```python
from build123d import *

# Parameters (mm, degrees)
ESQUISSE1_W        = 100
ESQUISSE1_H        = 100
ESQUISSE1_R        = 1.6
BOSS_EXTRU_1_DEPTH = 1.6
ESQUISSE2_R        = 5
BOSS_EXTRU_2_DEPTH = 20
ESQUISSE3_W        = 27.619166331
ESQUISSE3_H        = 14.436937143
BOSS_EXTRU_3_DEPTH = 15


with BuildPart() as part:
    # Esquisse1 → Boss.-Extru.1 (new body)
    with BuildSketch(Plane.XY):
        Rectangle(ESQUISSE1_W, ESQUISSE1_H)
        with Locations((-46, 46)):
            Circle(ESQUISSE1_R, mode=Mode.SUBTRACT)
        with Locations((46, 46)):
            Circle(ESQUISSE1_R, mode=Mode.SUBTRACT)
        with Locations((46, 4)):
            Circle(ESQUISSE1_R, mode=Mode.SUBTRACT)
        with Locations((-46, 4)):
            Circle(ESQUISSE1_R, mode=Mode.SUBTRACT)
        with Locations((-46, -46)):
            Circle(ESQUISSE1_R, mode=Mode.SUBTRACT)
        with Locations((46, -46)):
            Circle(ESQUISSE1_R, mode=Mode.SUBTRACT)
    extrude(amount=BOSS_EXTRU_1_DEPTH)

    # Esquisse2 → Boss.-Extru.2 (add)
    with BuildSketch(Plane.XY.offset(1.6)):
        with Locations((-26.099103373, -42.842866213)):
            Circle(ESQUISSE2_R)
        with Locations((-10.063114572, -42.842866213)):
            Circle(ESQUISSE2_R)
        with Locations((41.376738419, -34.563702957)):
            Circle(ESQUISSE2_R)
    extrude(amount=BOSS_EXTRU_2_DEPTH)

    # Esquisse3 → Boss.-Extru.3 (add)
    with BuildSketch(Plane.XY.offset(1.6)):
        with Locations((-34.191305716, 27.512141018)):
            Rectangle(ESQUISSE3_W, ESQUISSE3_H)
    extrude(amount=BOSS_EXTRU_3_DEPTH)


solid = part.part
```
Input: part model. Units: mm. Frame: model coordinates. A direction names the side the tool comes from. Give positions to 0.01 mm unless a question says otherwise; leave off trailing zeros. Order: outer loops, then holes, each group sorted by start corner. A loop starts at its lowest first (then second) coordinate and runs counter-clockwise, first axis right, second up.
1. Reachability of faces 5 (the cylindrical face through (36.38, -34.34, 11.46)), 6 (the flat face through (-34, 28, 16.6)), 7 (the flat face through (-20.382, 27, 9)), 8 (the flat face through (-34, 20.294, 9)) from +Z, -Z, +X, -X, +Y, -Y: full face, straight path, thin tool, end or side. Return the list, or none.
Derived:
face 5: +Z
face 6: +Z, +X, -X, +Y
face 7: +Z, +X, +Y, -Y
face 8: +Z, +X, -X
2. Mould query, pull axis Y, two halves, no side actions, for faces 1 (the flat face through (-34, 34.731, 9)), 2 (the flat face through (-48.001, 27, 9)), 3 (the cylindrical face through (-7.8, -47.3, 11.5)), 4 (the cylindrical face through (-27.183, -47.724, 11.46)). Classes: released by +Y, released by -Y, zero draft, split by the parting line, or undercut.
Derived:
face 1: released by +Y
face 2: zero draft
face 3: split by the parting line
face 4: undercut
3. Section A-A on y = 46. Return the cut outline in (x, z), and give its area (3 significant figures).
Derived:
outline: (-50, 0) - (-47.6, 0) - (-47.6, 1.6) - (-50, 1.6) - close; (-44.4, 0) - (44.4, 0) - (44.4, 1.6) - (-44.4, 1.6) - close; (47.6, 0) - (50, 0) - (50, 1.6) - (47.6, 1.6) - close
area: 150 mm2
4. Section D-D on z = 5. Return the cut outline in (x, y).
Derived:
outline: (-48, 20.29) - (-20.38, 20.29) - (-20.38, 34.73) - (-48, 34.73) - close; circle Ø10 at (-26.1, -42.84); circle Ø10 at (-10.06, -42.84); circle Ø10 at (41.38, -34.56)
5. Pin query (flat end, axial travel): pin 1 (3.5 mm diameter, centred on x = -46, y = 46, fed in from +Z); pin 2 (10 mm diameter, centred on y = -23.5, z = 7, fed in from +X); pin 3 (16 mm diameter, centred on x = -38, y = 28.5, fed in from +Z); pin 4 (12 mm diameter, centred on x = -30.5, z = 9, fed in from +Y). Return the tip coordinate at first contact, or that it passes through.
Derived:
pin 1: stops at z = 1.6
pin 2: passes through
pin 3: stops at z = 16.6
pin 4: stops at y = 34.73
6. Section C-C on y = 33.5. Return the cut outline in (x, z).
Derived:
outline: (-50, 0) - (50, 0) - (50, 1.6) - (-20.38, 1.6) - (-20.38, 16.6) - (-48, 16.6) - (-48, 1.6) - (-50, 1.6) - close
7. Section B-B on x = -46. Return the cut outline in (y, z).
Derived:
outline: (-50, 0) - (-47.6, 0) - (-47.6, 1.6) - (-50, 1.6) - close; (-44.4, 0) - (2.4, 0) - (2.4, 1.6) - (-44.4, 1.6) - close; (5.6, 0) - (44.4, 0) - (44.4, 1.6) - (34.73, 1.6) - (34.73, 16.6) - (20.29, 16.6) - (20.29, 1.6) - (5.6, 1.6) - close; (47.6, 0) - (50, 0) - (50, 1.6) - (47.6, 1.6) - close
8. Material intervals for L1, parallel to Y at x = 46, z = 0.6; L2, parallel to Z at x = -4, y = -38; L3, parallel to X at y = 29, z = 7.5, sorted ascending.
Derived:
L1: y = -50 to -47.6, -44.4 to 2.4, 5.6 to 44.4, 47.6 to 50
L2: z = 0 to 1.6
L3: x = -48 to -20.38
